Model file for the job. Use its own axes, mm. Face numbers are marked on the shaded views. A direction names the side the tool comes from. Coordinates: 2 decimals unless noted, no trailing zeros. Order: outer loops, then holes, each group sorted by start corner. A loop starts at its lowest first (then second) coordinate and runs counter-clockwise, first axis right, second up.
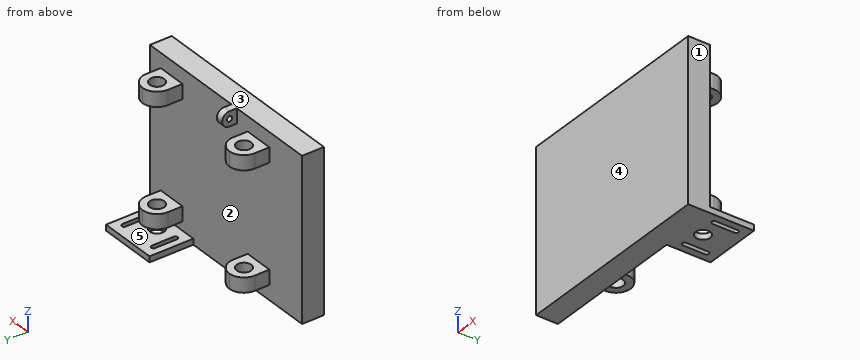
from build123d import *

# Parameters (mm, degrees)
SKETCH1_W               = 177.8
SKETCH1_H               = 139.7
BOSS_EXTRUDE1_DEPTH     = 19.05
SKETCH3_W               = 25.4
SKETCH3_H               = 12.7
BOSS_EXTRUDE2_DEPTH     = 25.4
SKETCH5_W               = 50.8
SKETCH5_H               = 5.08
BOSS_EXTRUDE3_DEPTH     = 38.1
CUT_EXTRUDE1_DEPTH      = 156.672163536
CUT_EXTRUDE1_DEPTH_BACK = 156.672163536
SKETCH4_R               = 6.35
CUT_EXTRUDE2_REACH      = 177.173
SKETCH7_W               = 6.35
SKETCH7_H               = 12.7
BOSS_EXTRUDE4_DEPTH     = 12.7
FILLET1_R               = 12.7
CUT_EXTRUDE3_REACH      = 133.216
SKETCH8_R               = 2.280315524
FILLET2_R               = 6.35


with BuildPart() as part:
    # Sketch1 → Boss-Extrude1 (new body)
    with BuildSketch(Plane(origin=(0, 0, 0), x_dir=(1, 0, 0), z_dir=(0, 1, 0))):
        Rectangle(SKETCH1_W, SKETCH1_H)
    extrude(amount=BOSS_EXTRUDE1_DEPTH)

    # Sketch3 → Boss-Extrude2 (add)
    with BuildSketch(Plane(origin=(0, 19.05, 0), x_dir=(1, 0, 0), z_dir=(0, 1, 0))):
        with Locations((-38.1, 50.8)):
            Rectangle(SKETCH3_W, SKETCH3_H)
        with Locations((63.5, 50.8)):
            Rectangle(SKETCH3_W, SKETCH3_H)
        with Locations((-38.1, -50.8)):
            Rectangle(SKETCH3_W, SKETCH3_H)
        with Locations((63.5, -50.8)):
            Rectangle(SKETCH3_W, SKETCH3_H)
    extrude(amount=BOSS_EXTRUDE2_DEPTH)

    # Sketch5 → Boss-Extrude3 (add)
    with BuildSketch(Plane(origin=(0, 19.05, 0), x_dir=(1, 0, 0), z_dir=(0, 1, 0))):
        with Locations((63.5, 67.31)):
            Rectangle(SKETCH5_W, SKETCH5_H)
    extrude(amount=BOSS_EXTRUDE3_DEPTH)

    # Sketch4 → Cut-Extrude1 (cut, two sides: drawn at the far end of the back side and taken through both)
    with BuildSketch(Plane(origin=(0, 0, 44.45), x_dir=(-1, 0, 0), z_dir=(0, 0, -1)).offset(-CUT_EXTRUDE1_DEPTH_BACK)):
        with Locations((38.1, 31.75)):
            Circle(SKETCH4_R)
        with Locations((-63.5, 31.75)):
            Circle(SKETCH4_R)
    extrude(amount=CUT_EXTRUDE1_DEPTH + CUT_EXTRUDE1_DEPTH_BACK, mode=Mode.SUBTRACT)

    # Sketch6 → Cut-Extrude2 (cut, up to next)
    with BuildSketch(Plane(origin=(0, 0, -69.85), x_dir=(-1, 0, 0), z_dir=(0, 0, -1)), mode=Mode.PRIVATE) as cut_extrude2_sk1:
        with BuildLine():
            Line((-48.25, 28.575), (-48.25, 47.625))
            ThreePointArc((-48.25, 47.625), (-46.25, 49.625), (-44.25, 47.625))
            Line((-44.25, 47.625), (-44.25, 28.575))
            ThreePointArc((-44.25, 28.575), (-46.25, 26.575), (-48.25, 28.575))
        make_face()
    cut_extrude2_tool1 = extrude(cut_extrude2_sk1.sketch, amount=-CUT_EXTRUDE2_REACH, mode=Mode.PRIVATE) & part.part
    # Sketch6 → Cut-Extrude2 (cut, up to next)
    with BuildSketch(Plane(origin=(0, 0, -69.85), x_dir=(-1, 0, 0), z_dir=(0, 0, -1)), mode=Mode.PRIVATE) as cut_extrude2_sk2:
        with BuildLine():
            Line((-82.75, 28.575), (-82.75, 47.625))
            ThreePointArc((-82.75, 47.625), (-80.75, 49.625), (-78.75, 47.625))
            Line((-78.75, 47.625), (-78.75, 28.575))
            ThreePointArc((-78.75, 28.575), (-80.75, 26.575), (-82.75, 28.575))
        make_face()
    cut_extrude2_tool2 = extrude(cut_extrude2_sk2.sketch, amount=-CUT_EXTRUDE2_REACH, mode=Mode.PRIVATE) & part.part
    add(cut_extrude2_tool1.solids().sort_by_distance((46.25, 38.1, -69.85))[0], mode=Mode.SUBTRACT)
    add(cut_extrude2_tool2.solids().sort_by_distance((80.75, 38.1, -69.85))[0], mode=Mode.SUBTRACT)

    # Sketch7 → Boss-Extrude4 (add)
    with BuildSketch(Plane(origin=(0, 19.05, 0), x_dir=(1, 0, 0), z_dir=(0, 1, 0))):
        with Locations((-9.525, -63.5)):
            Rectangle(SKETCH7_W, SKETCH7_H)
    extrude(amount=BOSS_EXTRUDE4_DEPTH)

    # Fillet1
    fillet1_edges = [part.edges().sort_by_distance(p)[0] for p in [
        (76.2, 44.45, -50.8),
        (50.8, 44.45, -50.8),
        (76.2, 44.45, 50.8),
        (50.8, 44.45, 50.8),
        (-25.4, 44.45, 50.8),
        (-50.8, 44.45, 50.8),
        (-25.4, 44.45, -50.8),
        (-50.8, 44.45, -50.8),
    ]]
    fillet(fillet1_edges, radius=FILLET1_R - 0.0001)  # a hair under: the kernel refuses the full size

    # Sketch8 → Cut-Extrude3 (cut, up to next)
    with BuildSketch(Plane(origin=(-6.35, 0, 0), x_dir=(0, 0, -1), z_dir=(1, 0, 0)), mode=Mode.PRIVATE) as cut_extrude3_sk1:
        with Locations((-63.5, 25.4)):
            Circle(SKETCH8_R)
    cut_extrude3_tool1 = extrude(cut_extrude3_sk1.sketch, amount=-CUT_EXTRUDE3_REACH, mode=Mode.PRIVATE) & part.part
    add(cut_extrude3_tool1.solids().sort_by_distance((-6.35, 25.4, 63.5))[0], mode=Mode.SUBTRACT)

    # Fillet2
    fillet2_edges = [part.edges().sort_by_distance(p)[0] for p in [
        (-9.525, 31.75, 57.15),
        (-9.525, 31.75, 69.85),
    ]]
    fillet(fillet2_edges, radius=FILLET2_R - 0.0001)  # a hair under: the kernel refuses the full size


solid = part.part
Q1. Cut at D-D, the plane x = -34. List the corners of the cut face in (y, z), plus the area to 3 significant figures.
Established:
outline: (0, -69.85) - (19.05, -69.85) - (19.05, -57.15) - (26.9, -57.15) - (26.9, -44.45) - (19.05, -44.45) - (19.05, 44.45) - (26.9, 44.45) - (26.9, 57.15) - (19.05, 57.15) - (19.05, 69.85) - (0, 69.85) - close; (36.6, -57.15) - (43.77, -57.15) - (43.77, -44.45) - (36.6, -44.45) - close; (36.6, 44.45) - (43.77, 44.45) - (43.77, 57.15) - (36.6, 57.15) - close
area: 3,040 mm2
Q2. Which spindle directions (+Z, -Z, +X, -X, +Y, -Y) get a long thin tool onto all of the face, cutting with end or side? Do the marked faces 4 and 5. Say none if no direction does.
Established:
face 4: +Z, -Z, +X, -X, -Y
face 5: +X, -X, +Y
Q3. Probe line 1 (X direction, y = 31.75, z = -48.5); line 2 (X direction, y = 22, z = 44.5); line 3 (Z direction, x = -28, y = 29). List the from-to ranges inside material, lowest first.
Established:
line 1: x = -50.8 to -44.45, -31.75 to -25.4, 50.8 to 57.15, 69.85 to 76.2
line 2: x = -50.8 to -25.4, 50.8 to 76.2
line 3: z = -57.15 to -44.45, 44.45 to 57.15
Q4. Mould opens along Z. For the marked faces 1, 2 and 3 say: pulls with the +Z half, pulls with the -Z half, needs draft (parallel to the pull), parting line crosses it, or undercut.
Established:
face 1: needs draft
face 2: undercut
face 3: pulls with the +Z half
Q5. Drop flat-ended pins along their axis: P1, Ø5.5, axis at y = 35, z = -67.5, coming from the -X side; P2, Ø10, axis at y = 27.5, z = 63, coming from the +X side; P3, Ø12.5, axis at x = -40.5, y = 28, coming from the +Z side. Give the stop position or say it passes through.
Established:
P1: stops at x = 38.1
P2: stops at x = -6.35
P3: stops at z = 57.15
Q6. Cut at A-A, the plane x = 80.75. List the corners of the cut face in (y, z) (3 decimals), plus the area to 3 significant figures.
Established:
outline: (0, -69.85) - (26.575, -69.85) - (26.575, -64.77) - (19.05, -64.77) - (19.05, 69.85) - (0, 69.85) - close; (49.625, -69.85) - (57.15, -69.85) - (57.15, -64.77) - (49.625, -64.77) - close
area: 2,740 mm2
Q7. Cut at C-C, the plane z = -54.5. Count the separate pieces of the cut face and the enclosed holes in it, plus the area to 3 significant figures.
Established:
separate pieces: 1
enclosed holes: 2
area: 4,290 mm2
